Autodesk Inventor part; units mm, degrees
ref_plane "YZ Plane" through (0, 0, 0) normal (1, 0, 0) x (0, 1, 0)
ref_plane "XZ Plane" through (0, 0, 0) normal (0, 1, 0) x (-1, 0, 0)
ref_plane "XY Plane" through (0, 0, 0) normal (0, 0, 1) x (1, 0, 0)
sketch "Sketch1" plane through (0, 0, 0) normal (0, 0, 1) x (1, 0, 0)
  line L0 (3.6, -8) -> (3.6, 8)
  line L1 (-3.6, 8) -> (-3.6, -8)
  arc A0 (3.6, 8) -> (-3.6, 8) centre (0, 8) ccw
  circle A1 centre (0, 8) radius 2.4
  circle A2 centre (0, 8) radius 3.2
  circle A3 centre (0, 0) radius 3.2
  circle A4 centre (0, 0) radius 2.4
  line L2 (0, 0) -> (0, 8) construction
  line L3 (-2.8, 5.7373) -> (-2.8, 2.2627)
  line L4 (2.8, 5.7373) -> (2.8, 2.2627)
  arc A5 (-2.8, 5.7373) -> (2.8, 5.7373) centre (0, 8) ccw
  arc A6 (2.8, 2.2627) -> (-2.8, 2.2627) centre (0, 0) ccw
  arc A7 (-3.6, -8) -> (3.6, -8) centre (0, -8) ccw
  circle A8 centre (0, -8) radius 3.2
  circle A9 centre (0, -8) radius 2.4
  line L5 (0, 0) -> (0, -8) construction
  line L6 (-2.8, -2.2627) -> (-2.8, -5.7373)
  line L7 (2.8, -2.2627) -> (2.8, -5.7373)
  arc A10 (-2.8, -2.2627) -> (2.8, -2.2627) centre (0, 0) ccw
  arc A11 (2.8, -5.7373) -> (-2.8, -5.7373) centre (0, -8) ccw
  dimension "d8" = 4.8
  dimension "d9" = 6.4
  dimension "d32" = 7.2
  dimension "d34" = 8
  dimension "d36" = 0.8
extrude "Extrusion1" add sketch "Sketch1" along normal mid plane 8 contours A7 L1 A0 L0 | A2 | A3 | A5 L4 A6 L3 | A8 | A10 L7 A11 L6
sketch "Sketch6" plane through (0, 0, 4) normal (0, 0, 1) x (1, 0, 0)
  circle A0 centre (0, 0) radius 2.4
  circle A1 centre (0, 8) radius 2.4
  circle A2 centre (0, 0) radius 3.2
  circle A3 centre (0, 8) radius 3.2
  arc A4 (2.8, 2.2627) -> (-2.8, 2.2627) centre (0, 0) ccw
  line L0 (-2.8, 5.7373) -> (-2.8, 2.2627)
  arc A5 (-2.8, 5.7373) -> (2.8, 5.7373) centre (0, 8) ccw
  line L1 (2.8, 5.7373) -> (2.8, 2.2627)
  line L2 (-2.8, -2.2627) -> (-2.8, -5.7373)
  arc A6 (-2.8, -2.2627) -> (2.8, -2.2627) centre (0, 0) ccw
  arc A7 (2.8, -5.7373) -> (-2.8, -5.7373) centre (0, -8) ccw
  line L3 (2.8, -2.2627) -> (2.8, -5.7373)
  circle A8 centre (0, -8) radius 3.2
  circle A9 centre (0, -8) radius 2.4
extrude "Extrusion7" cut sketch "Sketch6" against normal blind 0.8 contours A2 | A3 | A8
extrude "Extrusion8" cut sketch "Sketch6" against normal blind 3.1 contours A4 L0 A5 L1 | A6 L3 A7 L2
mirror "Mirror1" about plane through (0, 0, 0) normal (0, 0, 1) of "Extrusion7", "Extrusion8"
fillet "Fillet1" radius 0.1 6 edges at (0, 11.6, 4) (3.6, 0, 4) (-3.6, 0, 4) (0, 11.6, -4) (-3.6, 0, -4) (3.6, 0, -4)
fillet "Fillet1" radius 0.4 16 edges at (-2.8, 2.2627, 2.45) (-2.8, 5.7373, 2.45) (2.8, 2.2627, 2.45) (2.8, 5.7373, 2.45) (2.8, 5.7373, -2.45) (2.8, 2.2627, -2.45) (-2.8, 2.2627, -2.45) (-2.8, 5.7373, -2.45) (-2.8, -2.2627, 2.45) (-2.8, -5.7373, 2.45) (2.8, -5.7373, 2.45) (2.8, -2.2627, 2.45) (2.8, -2.2627, -2.45) (2.8, -5.7373, -2.45) (-2.8, -5.7373, -2.45) (-2.8, -2.2627, -2.45)
equation "\"d8\" = tpd"
equation "\"d9\" = tsd"
equation "\"d32\" = tlad"
equation "\"d34\" = lu"
equation "\"d14\" = lu"
equation "\"d41\" = tsl"
equation "\"d45\" = lf"
equation "\"d46\" = tf"
properties part number "32523-Yellow" material "ABS Plastic"
CAD build for the part. Positions are in the model's coordinates, mm. A direction names the side the tool comes from. Round coordinates to 2 decimals unless told otherwise and drop trailing zeros. Order: outer loops, then holes, each group sorted by start corner. A loop starts at its lowest first (then second) coordinate and runs counter-clockwise, first axis right, second up. Notation, with made-up numbers: (51, 33) -> (57, 33) arc R26 ccw to (57, 61) -> close; hole circle Ø7 at (14, 40). An arc over 180 degrees is marked (long way). Write item = value, one per line. Start each with the question number.
(1) Pin check, flat tips, straight feed: P1, Ø4, axis at x = 0, y = -1, coming from the +Z side; P2, Ø4, axis at x = -3, z = -3, coming from the +Y side. Stop position of each tip, or through.
(2) Which spindle directions (+Z, -Z, +X, -X, +Y, -Y) get a long thin tool onto all of the face, cutting with end or side? Do faces 5 (the flat face through (2.8, -4, 2)), 6 (the flat face through (3, 2, 4)), 7 (the flat face through (0, -4, -0.9)). Say none if no direction does.
(3) Cut at A-A, the plane y = 0. List the corners of the cut face in (x, z), then the cut area to 3 significant figures.
(4) Cut at B-B, the plane z = -2.5. List the corners of the cut face in (x, y).
(5) Pull direction Y, two halves, no side cores. Call faces 1 (the flat face through (-2.8, -4, 2)), 2 (the cylindrical face through (0, 4.4, 2.5)), 3 (the flat face through (-3.6, 0, 0)), 4 (the cylindrical face through (0.1, 11.6, 0.1)): released by +Y, released by -Y, zero draft, split by the parting line, or undercut.
(6) Cut at C-C, the plane x = 0. State how many separate pieces and enclosed holes the cut face has, then the cut area to 3 significant figures.
(7) Probe line 1 (Y direction, x = 0, z = 3.4); line 2 (Y direction, x = -1, z = -2.5); line 3 (X direction, y = 8.25, z = 2.5). List the from-to ranges inside material, lowest first. Write a range as [from, to].
Model answer:
q1.P1 = 3.2
q1.P2 = 11.46
q2.face_5 = +Z
q2.face_6 = +Z, +X, -X, +Y, -Y
q2.face_7 = -Z
q3.outline = (-3.6, -3.9) arc R0.1 ccw to (-3.5, -4) -> (-3.2, -4) -> (-3.2, -3.2) -> (-2.4, -3.2) -> (-2.4, 3.2) -> (-3.2, 3.2) -> (-3.2, 4) -> (-3.5, 4) arc R0.1 ccw to (-3.6, 3.9) -> close; (2.4, -3.2) -> (3.2, -3.2) -> (3.2, -4) -> (3.5, -4) arc R0.1 ccw to (3.6, -3.9) -> (3.6, 3.9) arc R0.1 ccw to (3.5, 4) -> (3.2, 4) -> (3.2, 3.2) -> (2.4, 3.2) -> close
q3.area = 16.6 mm2
q4.outline = (-3.6, -8) arc R3.6 ccw to (3.6, -8) -> (3.6, 8) arc R3.6 ccw to (-3.6, 8) -> close; hole (-2.8, -4.8) arc R0.4 ccw to (-2.16, -5.12) arc R3.6 cw to (2.16, -5.12) arc R0.4 ccw to (2.8, -4.8) -> (2.8, -3.2) arc R0.4 ccw to (2.16, -2.88) arc R3.6 cw to (-2.16, -2.88) arc R0.4 ccw to (-2.8, -3.2) -> close; hole (-2.8, 3.2) arc R0.4 ccw to (-2.16, 2.88) arc R3.6 cw to (2.16, 2.88) arc R0.4 ccw to (2.8, 3.2) -> (2.8, 4.8) arc R0.4 ccw to (2.16, 5.12) arc R3.6 cw to (-2.16, 5.12) arc R0.4 ccw to (-2.8, 4.8) -> close; hole circle Ø4.8 at (0, -8); hole circle Ø4.8 at (0, 0); hole circle Ø4.8 at (0, 8)
q5.face_1 = undercut
q5.face_2 = undercut
q5.face_3 = zero draft
q5.face_4 = released by +Y
q6.separate_pieces = 4
q6.enclosed_holes = 0
q6.area = 52.8 mm2
q7.line_1 = [-11.6, -11.2], [-4.8, -4.4], [-3.6, -3.2], [3.2, 3.6], [4.4, 4.8], [11.2, 11.6]
q7.line_2 = [-11.46, -10.18], [-5.82, -4.54], [-3.46, -2.18], [2.18, 3.46], [4.54, 5.82], [10.18, 11.46]
q7.line_3 = [-3.59, -2.39], [2.39, 3.59]
